Could you check a few things on this drawing? It's one solid part, dimensions in mm from its lowest x, y, z. A direction names the side the tool comes from. Give positions to 0.01 mm unless a question says otherwise; leave off trailing zeros. Write each loop counter-clockwise with the first axis right and the second up, starting at its lowest first coordinate (ties: lowest second). Pieces come first, ordered by that corner, then holes. Notation, with made-up numbers: (42.5, 1) -> (88.5, 1) arc R24 ccw to (88.5, 33) -> close; hole circle Ø5 at (-6, 21). An arc over 180 degrees is marked (long way). Answer as CSV lines item,"result". Start each with the question number.
1. On a 3-axis mill with a long thin cutter (end or side, diameter ignored), from which of +Z, -Z, +X, -X, +Y, -Y can I reach the whole of each face in a straight line? I mean the marked faces 1 and 2. Say none if no direction works.
2. I need wall thicknesses on line 1 (X direction, y = 0.8, z = 10); line 2 (Y direction, x = 61.7, z = 10) (3 decimals); line 3 (X direction, y = 60, z = 7.5). Which ranges of each line are inside material? Lowest first, please. Write a range as [from, to].
3. If we section it at D-D on z = 15: Write out the boundary of the cut face in (x, y).
4. I'm going to push flat-ended pins straight in: P1, Ø2.5, axis at x = 62.5, z = 11.5, coming from the -Y side; P2, Ø1.8, axis at x = 42, z = 10, coming from the -Y side; P3, Ø1, axis at x = 38.5, z = 12.5, coming from the +Y side. Where does each tip first touch, or does it pass through?
5. If we section it at A-A on z = 10: Write out the boundary of the cut face in (x, y) (3 decimals).
6. If we section it at C-C on y = 24: Write out the boundary of the cut face in (x, z).
7. If we mould it in two halves opening along X, with no side actions, what happens to the marked faces 3, 4, 5 and 6? For each: pulls with the +X half, pulls with the -X half, needs draft (parallel to the pull), parting line crosses it, or undercut.
8. If we section it at B-B on x = 42: Write out the boundary of the cut face in (y, z).
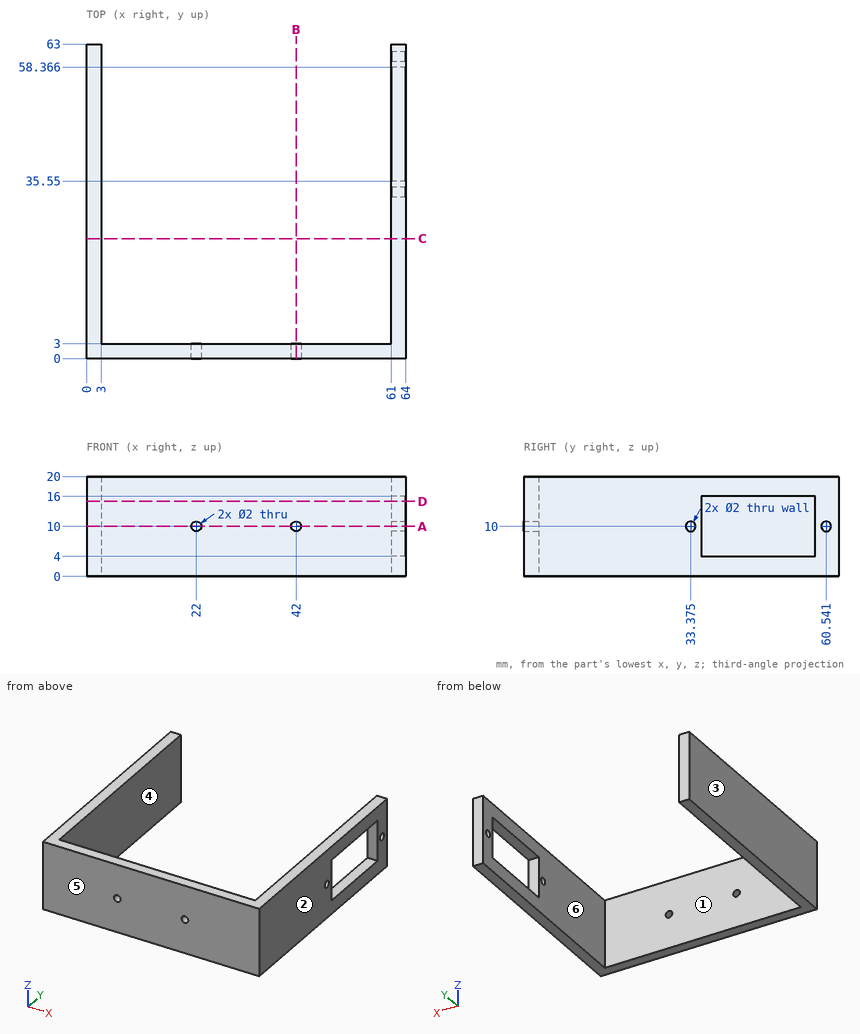
Computed values:
1,face 1,"+Z, -Z, +Y"
1,face 2,"+Z, -Z, +X, +Y, -Y"
2,line 1,"x = [0, 21], [23, 41], [43, 64]"
2,line 2,"y = [0, 32.375], [34.375, 35.55], [58.366, 59.541], [61.541, 63]"
2,line 3,"x = [0, 3], [61, 64]"
3,outline,"(0, 0) -> (64, 0) -> (64, 35.55) -> (61, 35.55) -> (61, 3) -> (3, 3) -> (3, 63) -> (0, 63) -> close; (61, 58.37) -> (64, 58.37) -> (64, 63) -> (61, 63) -> close"
4,P1,"stops at y = 0"
4,P2,"passes through"
4,P3,"stops at y = 3"
5,outline,"(0, 0) -> (21, 0) -> (21, 3) -> (3, 3) -> (3, 63) -> (0, 63) -> close; (23, 0) -> (41, 0) -> (41, 3) -> (23, 3) -> close; (43, 0) -> (64, 0) -> (64, 32.375) -> (61, 32.375) -> (61, 3) -> (43, 3) -> close; (61, 34.375) -> (64, 34.375) -> (64, 35.55) -> (61, 35.55) -> close; (61, 58.366) -> (64, 58.366) -> (64, 59.541) -> (61, 59.541) -> close; (61, 61.541) -> (64, 61.541) -> (64, 63) -> (61, 63) -> close"
6,outline,"(0, 0) -> (3, 0) -> (3, 20) -> (0, 20) -> close; (61, 0) -> (64, 0) -> (64, 20) -> (61, 20) -> close"
7,face 3,"pulls with the -X half"
7,face 4,"undercut"
7,face 5,"needs draft"
7,face 6,"undercut"
8,outline,"(0, 0) -> (3, 0) -> (3, 9) -> (0, 9) -> close; (0, 11) -> (3, 11) -> (3, 20) -> (0, 20) -> close"
